Verification items for this drawing (mm, ordinates from the low corner). Round coordinates to 2 decimals unless told otherwise and drop trailing zeros. Loops run counter-clockwise (first coordinate to the right, second up) from the corner with the lowest first, then second, coordinate; pieces in that order, holes last. Notation, with made-up numbers: M -7.5,13 L 1.5,13 A6 cw 1.5,17 Z; hole C 69.25,-10.75 d9. An arc over 180 degrees is marked long. Write item = value, one per line. Start each with the question number.
(1) Scan lines: L1, parallel to X at y = 1.5, z = 51; L2, parallel to Z at x = 32.5, y = 1.45; L3, parallel to X at y = 1.85, z = 76.5. Record each from-to range of solid material in increasing order. Write a range as from..to.
(2) Cross-section at A-A on x = 32.5. Record the boundary of the cut face in (y, z), plus the area to 3 significant figures.
(3) Cross-section at B-B on z = 51. Record the boundary of the cut face in (x, y).
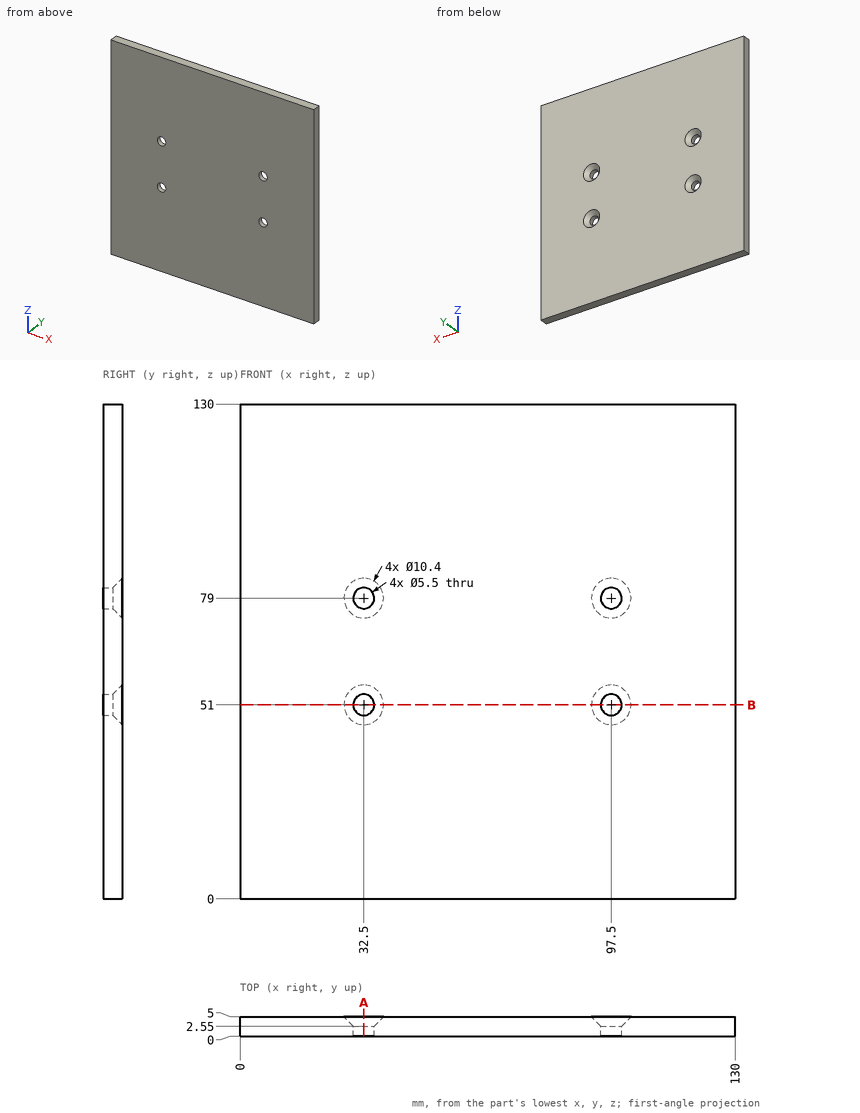
Result:
q1.L1 = 0..29.75, 35.25..94.75, 100.25..130
q1.L2 = 0..48.25, 53.75..76.25, 81.75..130
q1.L3 = 0..31.35, 33.65..96.35, 98.65..130
q2.outline = M 0,0 L 5,0 L 5,45.8 L 2.55,48.25 L 0,48.25 Z; M 0,53.75 L 2.55,53.75 L 5,56.2 L 5,73.8 L 2.55,76.25 L 0,76.25 Z; M 0,81.75 L 2.55,81.75 L 5,84.2 L 5,130 L 0,130 Z
q2.area = 583 mm^2
q3.outline = M 0,0 L 29.75,0 L 29.75,2.55 L 27.3,5 L 0,5 Z; M 35.25,0 L 94.75,0 L 94.75,2.55 L 92.3,5 L 37.7,5 L 35.25,2.55 Z; M 100.25,0 L 130,0 L 130,5 L 102.7,5 L 100.25,2.55 Z
